```python
from build123d import *

# Parameters (mm, degrees)
BASE_FLANGE1_DEPTH       = 80
CUT_EXTRUDE1_DEPTH       = 94.429117517
M3_CLEARANCE_HOLE1_D     = 3.4
M3_CLEARANCE_HOLE1_DEPTH = 2
M3_CLEARANCE_HOLE1_TIP   = 1.021463052
M4_CLEARANCE_HOLE1_D     = 4.5
M4_CLEARANCE_HOLE1_DEPTH = 2
M4_CLEARANCE_HOLE1_TIP   = 1.351936393
M3_CLEARANCE_HOLE2_D     = 3.4
M3_CLEARANCE_HOLE2_DEPTH = 2
M3_CLEARANCE_HOLE2_TIP   = 1.021463052
FILLET1_R                = 5
FILLET2_R                = 1


# Sheet-metal steps are written as plain solids
with BuildPart() as part:
    # Sketch1 → Base-Flange1 (new body)
    with BuildSketch(Plane(origin=(0, 0, 0), x_dir=(0, 0, -1), z_dir=(1, 0, 0))):
        with BuildLine():
            Line((0, 0), (0, 8.343145751))
            ThreePointArc((0, 8.343145751), (0.30448187, 9.87387948), (1.171572875, 11.171572875))
            Line((1.171572875, 11.171572875), (15.828427125, 25.828427125))
            ThreePointArc((15.828427125, 25.828427125), (17.12612052, 26.69551813), (18.656854249, 27))
            Line((18.656854249, 27), (40, 27))
            Line((40, 27), (40, 25))
            Line((40, 25), (18.656854249, 25))
            ThreePointArc((18.656854249, 25), (17.891487385, 24.847759065), (17.242640687, 24.414213562))
            Line((17.242640687, 24.414213562), (2.585786438, 9.757359313))
            ThreePointArc((2.585786438, 9.757359313), (2.152240935, 9.108512615), (2, 8.343145751))
            Line((2, 8.343145751), (2, 0))
            Line((2, 0), (0, 0))
        make_face()
    extrude(amount=BASE_FLANGE1_DEPTH)

    # Sketch2 → Cut-Extrude1 (cut, through all)
    with BuildSketch(Plane(origin=(0, 27, 0), x_dir=(1, 0, 0), z_dir=(0, 1, 0))):
        Polygon((0, 24), (8, 20), (8, 0), (0, 0), align=None)
        Polygon((80, 0), (80, 24), (72, 20), (72, 0), align=None)
    extrude(amount=-CUT_EXTRUDE1_DEPTH, mode=Mode.SUBTRACT)

    # M3 Clearance Hole1
    with Locations(Plane.XY):
        with Locations((20, 5), (35, 5), (45, 5), (60, 5)):
            Hole(M3_CLEARANCE_HOLE1_D / 2, depth=M3_CLEARANCE_HOLE1_DEPTH)
            with Locations((0, 0, -(M3_CLEARANCE_HOLE1_DEPTH + M3_CLEARANCE_HOLE1_TIP / 2))):  # 118° drill point
                Cone(0, M3_CLEARANCE_HOLE1_D / 2, M3_CLEARANCE_HOLE1_TIP, mode=Mode.SUBTRACT)

    # M4 Clearance Hole1
    with Locations(Plane(origin=(0, 27, 0), x_dir=(1, 0, 0), z_dir=(0, 1, 0))):
        with Locations((25, 31.5), (55, 31.5)):
            Hole(M4_CLEARANCE_HOLE1_D / 2, depth=M4_CLEARANCE_HOLE1_DEPTH)
            with Locations((0, 0, -(M4_CLEARANCE_HOLE1_DEPTH + M4_CLEARANCE_HOLE1_TIP / 2))):  # 118° drill point
                Cone(0, M4_CLEARANCE_HOLE1_D / 2, M4_CLEARANCE_HOLE1_TIP, mode=Mode.SUBTRACT)

    # M3 Clearance Hole2
    with Locations(Plane(origin=(0, 27, 0), x_dir=(1, 0, 0), z_dir=(0, 1, 0))):
        with Locations((7, 32), (73, 32)):
            Hole(M3_CLEARANCE_HOLE2_D / 2, depth=M3_CLEARANCE_HOLE2_DEPTH)
            with Locations((0, 0, -(M3_CLEARANCE_HOLE2_DEPTH + M3_CLEARANCE_HOLE2_TIP / 2))):  # 118° drill point
                Cone(0, M3_CLEARANCE_HOLE2_D / 2, M3_CLEARANCE_HOLE2_TIP, mode=Mode.SUBTRACT)

    # Fillet1
    fillet1_edges = [part.edges().sort_by_distance(p)[0] for p in [
        (0, 26, -40),
        (80, 26, -24),
        (80, 26, -40),
        (0, 26, -24),
    ]]
    fillet(fillet1_edges, radius=FILLET1_R)

    # Fillet2
    fillet2_edges = [part.edges().sort_by_distance(p)[0] for p in [
        (72, 26, -20),
        (8, 26, -20),
    ]]
    fillet(fillet2_edges, radius=FILLET2_R)


solid = part.part
```
Build history of the part. All positions in model axes, mm. A direction names the side the tool comes from. Coordinates: 2 decimals unless noted, no trailing zeros. Write each loop counter-clockwise with the first axis right and the second up, starting at its lowest first coordinate (ties: lowest second). Pieces come first, ordered by that corner, then holes.
1. Pull direction X, two halves, no side cores. Call faces 1 (the flat face through (72, 15, -7)), 2 (the flat face through (39.55, 17.19, -10.02)), 3 (the cylindrical face through (23.79, 25.986, -33.397)), 4 (the cylindrical face through (18.43, 4.35, -1.01)): released by +X, released by -X, zero draft, split by the parting line, or undercut.
Answer block:
face 1: released by +X
face 2: zero draft
face 3: undercut
face 4: undercut
2. Drill centre lines: probe 1 along X at (y, z) = (25.8, -32); probe 2 along Z at (x, y) = (58.5, 1.5); probe 3 along Y at (x, z) = (68, -33.5). Where is each one in solid material? Low to high.
Answer block:
probe 1: x = 0 to 5.3, 8.7 to 22.81, 27.19 to 52.81, 57.19 to 71.3, 74.7 to 80
probe 2: z = -2 to 0
probe 3: y = 25 to 27
3. Band-saw the part on B-B, the plane x = 25. Give the cut face in (y, z).
Answer block:
outline: (0, -2) - (8.34, -2) arc R2 cw to (9.76, -2.59) - (24.41, -17.24) arc R2 cw to (25, -18.66) - (25, -29.25) - (27, -29.25) - (27, -18.66) arc R4 ccw to (25.83, -15.83) - (11.17, -1.17) arc R4 ccw to (8.34, 0) - (0, 0) - close; (25, -40) - (27, -40) - (27, -33.75) - (25, -33.75) - close
4. Drop flat-ended pins along their axis: pin 1 (4 mm diameter, centred on x = 66.5, z = -16, fed in from -Y); pin 2 (12 mm diameter, centred on x = 18.5, z = -13.5, fed in from -Y); pin 3 (5.5 mm diameter, centred on x = 60, y = 5, fed in from -Z); pin 4 (10 mm diameter, centred on y = 16.5, z = -18.5, fed in from -X). Give the stop position or say it passes through.
Answer block:
pin 1: stops at y = 21.17
pin 2: stops at y = 14.67
pin 3: stops at z = -2
pin 4: passes through
5. Band-saw the part on A-A, the plane y = 5. Give the cut face in (x, z), and give its area (3 significant figures).
Answer block:
outline: (8, -2) - (18.3, -2) - (18.3, 0) - (8, 0) - close; (21.7, -2) - (33.3, -2) - (33.3, 0) - (21.7, 0) - close; (36.7, -2) - (43.3, -2) - (43.3, 0) - (36.7, 0) - close; (46.7, -2) - (58.3, -2) - (58.3, 0) - (46.7, 0) - close; (61.7, -2) - (72, -2) - (72, 0) - (61.7, 0) - close
area: 101 mm2
6. 3-axis set-ups, long thin cutter, end or side, ignore diameter. For faces 5 (the flat face through (40, 4, 0)), 6 (the flat face through (40, 4, -2)): which of +Z, -Z, +X, -X, +Y, -Y reach the whole face in a straight line?
Answer block:
face 5: +Z, +X, -X, +Y, -Y
face 6: -Z, +X, -X, -Y
7. Band-saw the part on C-C, the plane x = 50. Give the cut face in (y, z).
Answer block:
outline: (0, -2) - (8.34, -2) arc R2 cw to (9.76, -2.59) - (24.41, -17.24) arc R2 cw to (25, -18.66) - (25, -40) - (27, -40) - (27, -18.66) arc R4 ccw to (25.83, -15.83) - (11.17, -1.17) arc R4 ccw to (8.34, 0) - (0, 0) - close
8. Band-saw the part on D-D, the plane x = 60. Give the cut face in (y, z), and give its area (3 significant figures).
Answer block:
outline: (0, -2) - (3.3, -2) - (3.3, 0) - (0, 0) - close; (6.7, -2) - (8.34, -2) arc R2 cw to (9.76, -2.59) - (24.41, -17.24) arc R2 cw to (25, -18.66) - (25, -40) - (27, -40) - (27, -18.66) arc R4 ccw to (25.83, -15.83) - (11.17, -1.17) arc R4 ccw to (8.34, 0) - (6.7, 0) - close
area: 103 mm2
